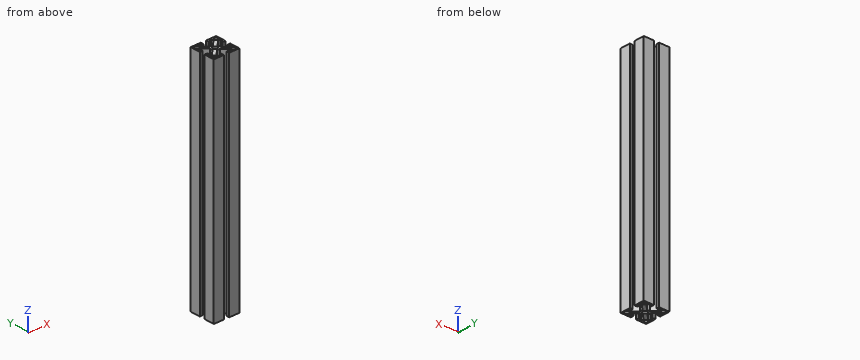
Autodesk Inventor part; units mm, degrees
ref_plane "Work Plane1" through (0, 0, 175) normal (0, 0, 1) x (1, 0, 0)
ref_plane "YZ Plane" through (0, 0, 0) normal (1, 0, 0) x (0, 1, 0)
ref_plane "XZ Plane" through (0, 0, 0) normal (0, 1, 0) x (-1, 0, 0)
sketch "Sketch1" plane through (0, 0, 0) normal (0, 0, 1) x (1, 0, 0)
  circle A0 centre (0, 0) radius 3.4
  line L0 (0, 0) -> (20, 20) construction
  line L1 (0, 0) -> (28.2843, 0) construction
  line L2 (20, 20) -> (4.15, 20)
  line L3 (4.15, 20) -> (4.15, 15.5)
  line L4 (4.15, 15.5) -> (7.1, 15.5)
  line L5 (7.1, 15.5) -> (7.1, 18)
  line L6 (7.1, 18) -> (10.25, 18)
  line L7 (10.25, 18) -> (10.25, 14)
  line L8 (0, 0) -> (0, 26.1056) construction
  line L9 (10.25, 14) -> (2.3, 6.05)
  line L10 (2.3, 6.05) -> (0, 6.05)
  circle A1 centre (15, 15) radius 3
  line L11 (20, 20) -> (20, 4.15)
  line L12 (20, 4.15) -> (15.5, 4.15)
  line L13 (15.5, 4.15) -> (15.5, 7.1)
  line L14 (15.5, 7.1) -> (18, 7.1)
  line L15 (18, 7.1) -> (18, 10.25)
  line L16 (18, 10.25) -> (14, 10.25)
  line L17 (14, 10.25) -> (6.05, 2.3)
  line L18 (6.05, 2.3) -> (6.05, 0)
  line L19 (-2.3, 6.05) -> (0, 6.05)
  line L20 (-10.25, 14) -> (-2.3, 6.05)
  line L21 (-10.25, 18) -> (-10.25, 14)
  line L22 (-4.15, 15.5) -> (-7.1, 15.5)
  line L23 (-7.1, 15.5) -> (-7.1, 18)
  line L24 (-7.1, 18) -> (-10.25, 18)
  line L25 (-4.15, 20) -> (-4.15, 15.5)
  line L26 (-20, 20) -> (-4.15, 20)
  circle A2 centre (-15, 15) radius 3
  line L27 (-20, 20) -> (-20, 4.15)
  line L28 (-14, 10.25) -> (-6.05, 2.3)
  line L29 (-18, 7.1) -> (-18, 10.25)
  line L30 (-18, 10.25) -> (-14, 10.25)
  line L31 (-20, 4.15) -> (-15.5, 4.15)
  line L32 (-15.5, 4.15) -> (-15.5, 7.1)
  line L33 (-15.5, 7.1) -> (-18, 7.1)
  line L34 (-6.05, 2.3) -> (-6.05, 0)
  line L35 (-6.05, -2.3) -> (-6.05, 0)
  line L36 (-14, -10.25) -> (-6.05, -2.3)
  line L37 (-18, -10.25) -> (-14, -10.25)
  line L38 (-15.5, -4.15) -> (-15.5, -7.1)
  line L39 (-15.5, -7.1) -> (-18, -7.1)
  line L40 (-18, -7.1) -> (-18, -10.25)
  line L41 (-20, -4.15) -> (-15.5, -4.15)
  line L42 (-20, -20) -> (-20, -4.15)
  circle A3 centre (-15, -15) radius 3
  line L43 (-20, -20) -> (-4.15, -20)
  line L44 (-10.25, -14) -> (-2.3, -6.05)
  line L45 (-7.1, -18) -> (-10.25, -18)
  line L46 (-10.25, -18) -> (-10.25, -14)
  line L47 (-4.15, -20) -> (-4.15, -15.5)
  line L48 (-4.15, -15.5) -> (-7.1, -15.5)
  line L49 (-7.1, -15.5) -> (-7.1, -18)
  line L50 (-2.3, -6.05) -> (0, -6.05)
  line L51 (2.3, -6.05) -> (0, -6.05)
  line L52 (10.25, -14) -> (2.3, -6.05)
  line L53 (10.25, -18) -> (10.25, -14)
  line L54 (4.15, -15.5) -> (7.1, -15.5)
  line L55 (7.1, -15.5) -> (7.1, -18)
  line L56 (7.1, -18) -> (10.25, -18)
  line L57 (4.15, -20) -> (4.15, -15.5)
  line L58 (20, -20) -> (4.15, -20)
  circle A4 centre (15, -15) radius 3
  line L59 (20, -20) -> (20, -4.15)
  line L60 (14, -10.25) -> (6.05, -2.3)
  line L61 (18, -7.1) -> (18, -10.25)
  line L62 (18, -10.25) -> (14, -10.25)
  line L63 (20, -4.15) -> (15.5, -4.15)
  line L64 (15.5, -4.15) -> (15.5, -7.1)
  line L65 (15.5, -7.1) -> (18, -7.1)
  line L66 (6.05, -2.3) -> (6.05, 0)
  point P0 (0, 6.05)
  point P1 (-6.05, 0)
  point P2 (0, -6.05)
  dimension "d0" = 6.8
  dimension "d1" = 45
  dimension "d2" = 20
  dimension "d3" = 6
  dimension "d4" = 15
  dimension "d5" = 10.25
  dimension "d6" = 7.1
  dimension "d7" = 4.15
  dimension "d8" = 4.5
  dimension "d9" = 2
  dimension "d10" = 13.95
  dimension "d11" = 6
  dimension "d14" = 360
extrude "Extrusion1" add sketch "Sketch1" along normal blind 350
ref_plane "Work Plane1" through (0, 0, 175) normal (0, 0, 1) x (1, 0, 0)
properties part number "Aluminum_Profile_4040_100.14mm_bottom" material "Aluminum 6061-AHC"
Source: CAD feature listing. Evaluate the final solid. Frame: model axes, mm. Give positions to 0.01 mm unless a question says otherwise; leave off trailing zeros. Use a Markdown table: item, result.
Q1. Material intervals for line 1 (Y direction, x = -15, z = 255); line 2 (X direction, y = 8, z = 269); line 3 (Y direction, x = 5, z = 276.5), sorted ascending. Write a range as [from, to].
A:
| item | result |
|---|---|
| line 1 | [-20, -18], [-12, -10.25], [10.25, 12], [18, 20] |
| line 2 | [-20, -18], [-11.75, -4.25], [4.25, 11.75], [18, 20] |
| line 3 | [-20, -15.5], [-8.75, 8.75], [15.5, 20] |
Q2. First-contact query: P1, Ø1.5, axis at y = 3, z = 123, coming from the +X side; P2, Ø5, axis at x = -0.5, z = 252.5, coming from the +Y side; P3, Ø1.4, axis at y = -1, z = 165.5, coming from the +X side. Flat tips, straight axial feed; report the tip coordinate or a pass-through.
A:
| item | result |
|---|---|
| P1 | x = 7.5 |
| P2 | y = 6.75 |
| P3 | x = 6.05 |
Q3. Section A-A (z = 317). State how many separate pieces and enclosed holes the cut face has, and give its area (3 significant figures).
A:
| item | result |
|---|---|
| separate pieces | 1 |
| enclosed holes | 5 |
| area | 716 mm^2 |
